from build123d import *

# Parameters (mm, degrees)
F0_W     = 5.8146030642
F0_H     = 3.8764025085
F1_DEPTH = 25.4


with BuildPart() as f1:
    # F0 (on Top) → F1 (new body)
    with BuildSketch(Plane.XY):
        with BuildLine():
            Line((60.0847271035, 0), (75.8325080935, 0))
            ThreePointArc((75.8325080935, 0), (75.8011270946, 2.1813791382), (75.7070100699, 4.3609528802))
            Line((75.7070100699, 4.3609528802), (59.9262590279, 4.3609528802))
            ThreePointArc((59.9262590279, 4.3609528802), (60.0450970152, 2.1819155663), (60.0847271035, 0))
        make_face()
        with BuildLine():
            ThreePointArc((5.8146030642, -75.6092565428), (55.6394878556, -51.524913148), (75.8325080935, 0))
            Line((75.8325080935, 0), (60.0847271035, 0))
            ThreePointArc((60.0847271035, 0), (60.0534252964, -1.939211508), (59.9595524891, -3.8764025085))
            ThreePointArc((59.9595524891, -3.8764025085), (43.1682524028, -41.793258016), (5.8146030642, -59.8027158439))
            Line((5.8146030642, -59.8027158439), (5.8146030642, -75.6092565428))
        make_face()
        with BuildLine():
            Line((59.9262590279, 4.3609528802), (75.7070100699, 4.3609528802))
            ThreePointArc((75.7070100699, 4.3609528802), (54.1343102449, 53.1041028364), (5.8146030642, 75.6092565428))
            Line((5.8146030642, 75.6092565428), (5.8146030642, 59.8027158439))
            ThreePointArc((5.8146030642, 59.8027158439), (42.9989826308, 41.9673911962), (59.9262590279, 4.3609528802))
        make_face()
        with BuildLine():
            ThreePointArc((0, -75.8325080935), (2.9094436775, -75.7766746515), (5.8146030642, -75.6092565428))
            Line((5.8146030642, -75.6092565428), (5.8146030642, -59.8027158439))
            ThreePointArc((5.8146030642, -59.8027158439), (2.9107189466, -60.0141828763), (0, -60.0847271035))
            Line((0, -60.0847271035), (0, -75.8325080935))
        make_face()
        with BuildLine():
            Line((5.8146030642, 0), (60.0847271035, 0))
            ThreePointArc((60.0847271035, 0), (60.0450970152, 2.1819155663), (59.9262590279, 4.3609528802))
            Line((59.9262590279, 4.3609528802), (5.8146030642, 4.3609528802))
            Line((5.8146030642, 4.3609528802), (0, 4.3609528802))
            Line((0, 4.3609528802), (0, 0))
            Line((0, 0), (5.8146030642, 0))
        make_face()
        with BuildLine():
            ThreePointArc((59.9595524891, -3.8764025085), (60.0534252964, -1.939211508), (60.0847271035, 0))
            Line((60.0847271035, 0), (5.8146030642, 0))
            Line((5.8146030642, 0), (5.8146030642, -3.8764025085))
            Line((5.8146030642, -3.8764025085), (59.9595524891, -3.8764025085))
        make_face()
        with BuildLine():
            Line((5.8146030642, 59.8027158439), (5.8146030642, 75.6092565428))
            ThreePointArc((5.8146030642, 75.6092565428), (2.9094436775, 75.7766746515), (0, 75.8325080935))
            Line((0, 75.8325080935), (0, 60.0847271035))
            ThreePointArc((0, 60.0847271035), (2.9107189466, 60.0141828763), (5.8146030642, 59.8027158439))
        make_face()
        with BuildLine():
            ThreePointArc((-4.3609519489, -75.7070101236), (-2.1813786719, -75.801127108), (0, -75.8325080935))
            Line((0, -75.8325080935), (0, -60.0847271035))
            ThreePointArc((0, -60.0847271035), (-2.1819150998, -60.0450970321), (-4.3609519489, -59.9262590956))
            Line((-4.3609519489, -59.9262590956), (-4.3609519489, -75.7070101236))
        make_face()
        with BuildLine():
            ThreePointArc((0, -60.0847271035), (2.9107189466, -60.0141828763), (5.8146030642, -59.8027158439))
            Line((5.8146030642, -59.8027158439), (5.8146030642, -3.8764025085))
            Line((5.8146030642, -3.8764025085), (0, -3.8764025085))
            Line((0, -3.8764025085), (0, -60.0847271035))
        make_face()
        with Locations((2.9073015321, -1.9382012542)):
            Rectangle(F0_W, F0_H)
        with BuildLine():
            Line((0, 60.0847271035), (0, 75.8325080935))
            ThreePointArc((0, 75.8325080935), (-2.1813786719, 75.801127108), (-4.3609519489, 75.7070101236))
            Line((-4.3609519489, 75.7070101236), (-4.3609519489, 59.9262590956))
            ThreePointArc((-4.3609519489, 59.9262590956), (-2.1819150998, 60.0450970321), (0, 60.0847271035))
        make_face()
        with BuildLine():
            Line((5.8146030642, 4.3609528802), (5.8146030642, 59.8027158439))
            ThreePointArc((5.8146030642, 59.8027158439), (2.9107189466, 60.0141828763), (0, 60.0847271035))
            Line((0, 60.0847271035), (0, 4.3609528802))
            Line((0, 4.3609528802), (5.8146030642, 4.3609528802))
        make_face()
        with BuildLine():
            ThreePointArc((-75.733366407, -3.8764025085), (-53.7929735729, -53.4498388953), (-4.3609519489, -75.7070101236))
            Line((-4.3609519489, -75.7070101236), (-4.3609519489, -59.9262590956))
            ThreePointArc((-4.3609519489, -59.9262590956), (-42.6576889746, -42.3142529468), (-59.9595524891, -3.8764025085))
            Line((-59.9595524891, -3.8764025085), (-75.733366407, -3.8764025085))
        make_face()
        with BuildLine():
            ThreePointArc((-4.3609519489, -59.9262590956), (-2.1819150998, -60.0450970321), (0, -60.0847271035))
            Line((0, -60.0847271035), (0, -3.8764025085))
            Line((0, -3.8764025085), (-4.3609519489, -3.8764025085))
            Line((-4.3609519489, -3.8764025085), (-4.3609519489, -59.9262590956))
        make_face()
        with BuildLine():
            Line((0, -3.8764025085), (0, 0))
            Line((0, 0), (0, 4.3609528802))
            Line((0, 4.3609528802), (0, 60.0847271035))
            ThreePointArc((0, 60.0847271035), (-2.1819150998, 60.0450970321), (-4.3609519489, 59.9262590956))
            Line((-4.3609519489, 59.9262590956), (-4.3609519489, 4.3609528802))
            Line((-4.3609519489, 4.3609528802), (-4.3609519489, 0))
            Line((-4.3609519489, 0), (-4.3609519489, -3.8764025085))
            Line((-4.3609519489, -3.8764025085), (0, -3.8764025085))
        make_face()
        with BuildLine():
            Line((-4.3609519489, 59.9262590956), (-4.3609519489, 75.7070101236))
            ThreePointArc((-4.3609519489, 75.7070101236), (-53.6216803775, 53.6216810371), (-75.7070100699, 4.3609528802))
            Line((-75.7070100699, 4.3609528802), (-59.9262590279, 4.3609528802))
            ThreePointArc((-59.9262590279, 4.3609528802), (-42.4863176505, 42.4863183108), (-4.3609519489, 59.9262590956))
        make_face()
        with BuildLine():
            ThreePointArc((-75.8325080935, 0), (-75.8077186201, -1.938835055), (-75.733366407, -3.8764025085))
            Line((-75.733366407, -3.8764025085), (-59.9595524891, -3.8764025085))
            ThreePointArc((-59.9595524891, -3.8764025085), (-60.0534252964, -1.939211508), (-60.0847271035, 0))
            Line((-60.0847271035, 0), (-75.8325080935, 0))
        make_face()
        with BuildLine():
            Line((-59.9262590279, 4.3609528802), (-75.7070100699, 4.3609528802))
            ThreePointArc((-75.7070100699, 4.3609528802), (-75.8011270946, 2.1813791382), (-75.8325080935, 0))
            Line((-75.8325080935, 0), (-60.0847271035, 0))
            ThreePointArc((-60.0847271035, 0), (-60.0450970152, 2.1819155663), (-59.9262590279, 4.3609528802))
        make_face()
        with BuildLine():
            ThreePointArc((-60.0847271035, 0), (-60.0534252964, -1.939211508), (-59.9595524891, -3.8764025085))
            Line((-59.9595524891, -3.8764025085), (-4.3609519489, -3.8764025085))
            Line((-4.3609519489, -3.8764025085), (-4.3609519489, 0))
            Line((-4.3609519489, 0), (-60.0847271035, 0))
        make_face()
        with BuildLine():
            Line((-4.3609519489, 4.3609528802), (-59.9262590279, 4.3609528802))
            ThreePointArc((-59.9262590279, 4.3609528802), (-60.0450970152, 2.1819155663), (-60.0847271035, 0))
            Line((-60.0847271035, 0), (-4.3609519489, 0))
            Line((-4.3609519489, 0), (-4.3609519489, 4.3609528802))
        make_face()
    extrude(amount=F1_DEPTH)


solid = f1.part
Work out the finished part from the listing and answer in its coordinate system (mm). A direction names the side the tool comes from. Give positions to 0.01 mm unless a question says otherwise; leave off trailing zeros. Loops run counter-clockwise (first coordinate to the right, second up) from the corner with the lowest first, then second, coordinate; pieces in that order, holes last. Notation, with made-up numbers: (53, -31.75) - (83, -31.75) arc R6 ccw to (83, -24.75) - close; hole circle Ø11 at (-14, 8). An arc over 180 degrees is marked (long way). Answer in a Markdown table with one row per item. Add a question column.
Q1. The part is cut by section D-D (y = -65.5). Determine the outline of the cut face in (x, z), and give its area (3 significant figures).
Q2. Each of these flat-tipped pins is pushed along its axis until it touches: P1, Ø7.5, axis at x = -44, z = 19, coming from the -Y side; P2, Ø8, axis at y = 15, z = 3, coming from the +X side; P3, Ø12, axis at y = 24, z = 13, coming from the +X side; P4, Ø3, axis at y = 1.5, z = 3.5, coming from the +X side. Where does it stop, or does it pass through?
Q3. The part is cut by section C-C (y = 24.5). Determine the outline of the cut face in (x, z), and give its area (3 significant figures).
Q4. Consider line 1 along X through (y, z) = (11.5, 10.75); line 2 along X through (y, z) = (-38, 19.75); line 3 along Y through (x, z) = (-31.5, 9.5). Determine where each line is inside the solid, lowest interval first.
Q5. The part is cut by section A-A (x = -46.5). Determine the outline of the cut face in (y, z), and give its area (3 significant figures).
Q6. Determine the mould class of faces 3 (the flat face through (5.815, -32, 13)), 4 (the flat face through (-1, 1, 25.4)) for opening direction X: released by +X, released by -X, zero draft, split by the parting line, or undercut.
Q7. The part is cut by section B-B (z = 7). Determine the outline of the cut face in (x, y).
Q8. A tool of negligible diameter and unlimited length cuts with its end or side. For faces 1 (the flat face through (-1, 1, 0)), 2 (the flat face through (33, -3.876, 13)), from which of +Z, -Z, +X, -X, +Y, -Y can it reach the whole face along a straight path? Write none if from no direction.
Solution:
| question | item | result |
|---|---|---|
| 1 | outline | (-38.21, 0) - (38.21, 0) - (38.21, 25.4) - (-38.21, 25.4) - close |
| 1 | area | 1,940 mm² |
| 2 | P1 | stops at y = -64.27 |
| 2 | P2 | stops at x = 75.03 |
| 2 | P3 | stops at x = 73.67 |
| 2 | P4 | stops at x = 75.83 |
| 3 | outline | (-71.77, 0) - (-54.86, 0) - (-54.86, 25.4) - (-71.77, 25.4) - close; (-4.36, 0) - (5.81, 0) - (5.81, 25.4) - (-4.36, 25.4) - close; (54.86, 0) - (71.77, 0) - (71.77, 25.4) - (54.86, 25.4) - close |
| 3 | area | 1,120 mm² |
| 4 | line 1 | x = -74.96 to -58.97, -4.36 to 5.81, 58.97 to 74.96 |
| 4 | line 2 | x = -65.62 to -46.54, -4.36 to 5.81, 46.54 to 65.62 |
| 4 | line 3 | y = -68.98 to -51.17, -3.88 to 4.36, 51.17 to 68.98 |
| 5 | outline | (-59.9, 0) - (-38.05, 0) - (-38.05, 25.4) - (-59.9, 25.4) - close; (-3.88, 0) - (4.36, 0) - (4.36, 25.4) - (-3.88, 25.4) - close; (38.05, 0) - (59.9, 0) - (59.9, 25.4) - (38.05, 25.4) - close |
| 5 | area | 1,320 mm² |
| 6 | face 3 | undercut |
| 6 | face 4 | zero draft |
| 7 | outline | circle Ø151.67 at (0, 0); hole (-59.96, -3.88) arc R60.08 ccw to (-4.36, -59.93) - (-4.36, -3.88) - close; hole (-59.93, 4.36) - (-4.36, 4.36) - (-4.36, 59.93) arc R60.08 ccw to start; hole (5.81, -59.8) arc R60.08 ccw to (59.96, -3.88) - (5.81, -3.88) - close; hole (5.81, 4.36) - (59.93, 4.36) arc R60.08 ccw to (5.81, 59.8) - close |
| 8 | face 1 | -Z, +X, -X, +Y, -Y |
| 8 | face 2 | +Z, -Z |
